```python
from build123d import *

# Parameters (mm, degrees)
SKETCH1_W                                         = 31.75
SKETCH1_H                                         = 160.3375
EXTRUDE1_DEPTH                                    = 62.70625
EXTRUDE2_DEPTH                                    = 107.616906566
EXTRUDE3_REACH                                    = 108.617
SKETCH15_W                                        = 3.96875
SKETCH15_H                                        = 9.525
EXTRUDE6_DEPTH                                    = 173.893618507
CUT_EXTRUDE1_DEPTH                                = 107.616906566
SKETCH17_W                                        = 1.5875
SKETCH17_H                                        = 19.177
CUT_EXTRUDE2_DEPTH                                = 96.8375
CBORE_FOR_1_4_SOCKET_HEAD_CAP_SCREW4_D            = 6.7564
CBORE_FOR_1_4_SOCKET_HEAD_CAP_SCREW4_CBORE_D      = 11.1125
CBORE_FOR_1_4_SOCKET_HEAD_CAP_SCREW4_CBORE_DEPTH  = 6.35
CBORE_FOR_5_16_SOCKET_HEAD_CAP_SCREW2_D           = 8.4328
CBORE_FOR_5_16_SOCKET_HEAD_CAP_SCREW2_DEPTH       = 15.875
CBORE_FOR_5_16_SOCKET_HEAD_CAP_SCREW2_CBORE_D     = 13.49502
CBORE_FOR_5_16_SOCKET_HEAD_CAP_SCREW2_CBORE_DEPTH = 7.9375
CBORE_FOR_5_16_SOCKET_HEAD_CAP_SCREW3_D           = 8.4328
CBORE_FOR_5_16_SOCKET_HEAD_CAP_SCREW3_CBORE_D     = 13.49502
CBORE_FOR_5_16_SOCKET_HEAD_CAP_SCREW3_CBORE_DEPTH = 7.9375
CBORE_FOR_1_4_SOCKET_HEAD_CAP_SCREW2_D            = 6.7564
CBORE_FOR_1_4_SOCKET_HEAD_CAP_SCREW2_CBORE_D      = 11.1125
CBORE_FOR_1_4_SOCKET_HEAD_CAP_SCREW2_CBORE_DEPTH  = 6.35
FILLET1_R                                         = 3.175
SKETCH32_R                                        = 6.35
CUT_EXTRUDE7_DEPTH                                = 22.225
CUT_EXTRUDE8_START                                = 22.225
SKETCH33_R                                        = 6.35
CUT_EXTRUDE8_DEPTH                                = 22.225
SKETCH41_W                                        = 19.05
SKETCH41_H                                        = 25.520262047
CUT_EXTRUDE9_DEPTH                                = 19.05
SKETCH43_W                                        = 6.35
SKETCH43_H                                        = 38.0746
CUT_EXTRUDE11_DEPTH                               = 22.225
CUT_EXTRUDE12_DEPTH                               = 7.14375
CBORE_FOR_1_4_SOCKET_HEAD_CAP_SCREW5_D            = 6.7564
CBORE_FOR_1_4_SOCKET_HEAD_CAP_SCREW5_CBORE_D      = 11.1125
CBORE_FOR_1_4_SOCKET_HEAD_CAP_SCREW5_CBORE_DEPTH  = 9.525
FILLET2_R                                         = 3.175
FILLET3_R                                         = 3.175
CUT_EXTRUDE13_DEPTH                               = 173.893618516
CUT_EXTRUDE14_DEPTH                               = 38.1
FILLET4_R                                         = 3.175


with BuildPart() as part:
    # Sketch1 → Extrude1 (new, symmetric)
    with BuildSketch(Plane.XY):
        Rectangle(SKETCH1_W, SKETCH1_H)
    extrude(amount=EXTRUDE1_DEPTH, both=True)

    # Sketch2 → Extrude2 (cut, through all)
    with BuildSketch(Plane(origin=(15.875, 0, 0), x_dir=(0, 0, -1), z_dir=(1, 0, 0))):
        Polygon((-62.70625, -80.16875), (-61.542285786, -35.71875), (-61.542285786, 80.16875), (-62.70625, 80.16875), align=None)
        Polygon((62.70625, -80.16875), (61.542285786, -35.71875), (61.542285786, 80.16875), (62.70625, 80.16875), align=None)
    extrude(amount=-EXTRUDE2_DEPTH, mode=Mode.SUBTRACT)

    # Sketch3 → Extrude3 (cut, up to next)
    with BuildSketch(Plane(origin=(15.875, 0, 0), x_dir=(0, 0, -1), z_dir=(1, 0, 0)), mode=Mode.PRIVATE) as extrude3_sk1:
        with BuildLine():
            Line((-19.0373, -59.53125), (-19.0373, -50.00625))
            ThreePointArc((-19.0373, -50.00625), (-19.96723597, -47.76118597), (-22.2123, -46.83125))
            Line((-22.2123, -46.83125), (-33.5788, -46.83125))
            ThreePointArc((-33.5788, -46.83125), (-41.5163, -38.89375), (-49.4538, -46.83125))
            Line((-49.4538, -46.83125), (-49.4538, -67.46875))
            ThreePointArc((-49.4538, -67.46875), (-41.5163, -75.40625), (-33.5788, -67.46875))
            Line((-33.5788, -67.46875), (-33.5788, -62.70625))
            Line((-33.5788, -62.70625), (-22.2123, -62.70625))
            ThreePointArc((-22.2123, -62.70625), (-19.96723597, -61.77631403), (-19.0373, -59.53125))
        make_face()
    extrude3_tool1 = extrude(extrude3_sk1.sketch, amount=-EXTRUDE3_REACH, mode=Mode.PRIVATE) & part.part
    # Sketch3 → Extrude3 (cut, up to next)
    with BuildSketch(Plane(origin=(15.875, 0, 0), x_dir=(0, 0, -1), z_dir=(1, 0, 0)), mode=Mode.PRIVATE) as extrude3_sk2:
        with BuildLine():
            Line((49.4538, -67.46875), (49.4538, -46.83125))
            ThreePointArc((49.4538, -46.83125), (41.5163, -38.89375), (33.5788, -46.83125))
            Line((33.5788, -46.83125), (22.2123, -46.83125))
            ThreePointArc((22.2123, -46.83125), (19.96723597, -47.76118597), (19.0373, -50.00625))
            Line((19.0373, -50.00625), (19.0373, -59.53125))
            ThreePointArc((19.0373, -59.53125), (19.96723597, -61.77631403), (22.2123, -62.70625))
            Line((22.2123, -62.70625), (33.5788, -62.70625))
            Line((33.5788, -62.70625), (33.5788, -67.46875))
            ThreePointArc((33.5788, -67.46875), (41.5163, -75.40625), (49.4538, -67.46875))
        make_face()
    extrude3_tool2 = extrude(extrude3_sk2.sketch, amount=-EXTRUDE3_REACH, mode=Mode.PRIVATE) & part.part
    add(extrude3_tool1.solids().sort_by_distance((15.875, -56.432782, 36.973416))[0], mode=Mode.SUBTRACT)
    add(extrude3_tool2.solids().sort_by_distance((15.875, -56.432782, -36.973416))[0], mode=Mode.SUBTRACT)

    # Sketch15 → Extrude6 (cut, through all)
    with BuildSketch(Plane(origin=(0, 80.16875, 0), x_dir=(1, 0, 0), z_dir=(0, 1, 0))):
        with Locations((13.890625, -22.621875)):
            Rectangle(SKETCH15_W, SKETCH15_H)
        with Locations((13.890625, 22.621875)):
            Rectangle(SKETCH15_W, SKETCH15_H)
    extrude(amount=-EXTRUDE6_DEPTH, mode=Mode.SUBTRACT)

    # Sketch16 → Cut-Extrude1 (cut, through all)
    with BuildSketch(Plane(origin=(15.875, 0, 0), x_dir=(0, 0, -1), z_dir=(1, 0, 0))):
        with BuildLine():
            Line((-45.667285786, 80.16875), (45.667285786, 80.16875))
            Line((45.667285786, 80.16875), (45.667285786, -23.01875))
            ThreePointArc((45.667285786, -23.01875), (43.807413847, -27.508878061), (39.317285786, -29.36875))
            Line((39.317285786, -29.36875), (-39.317285786, -29.36875))
            ThreePointArc((-39.317285786, -29.36875), (-43.807413847, -27.508878061), (-45.667285786, -23.01875))
            Line((-45.667285786, -23.01875), (-45.667285786, 80.16875))
        make_face()
    extrude(amount=-CUT_EXTRUDE1_DEPTH, mode=Mode.SUBTRACT)

    # Sketch17 → Cut-Extrude2 (cut, symmetric)
    with BuildSketch(Plane.XY):
        with Locations((-15.08125, -70.58025)):
            Rectangle(SKETCH17_W, SKETCH17_H)
    extrude(amount=CUT_EXTRUDE2_DEPTH, both=True, mode=Mode.SUBTRACT)

    # CBORE for 1/4 Socket Head Cap Screw4 (through all)
    with Locations(Plane(origin=(15.875, 0, 0), x_dir=(0, 0, -1), z_dir=(1, 0, 0))):
        with Locations((-56.35625, -70.58025), (56.35625, -70.58025), (0, -70.58025)):
            CounterBoreHole(CBORE_FOR_1_4_SOCKET_HEAD_CAP_SCREW4_D / 2, CBORE_FOR_1_4_SOCKET_HEAD_CAP_SCREW4_CBORE_D / 2, CBORE_FOR_1_4_SOCKET_HEAD_CAP_SCREW4_CBORE_DEPTH)

    # CBORE for 5/16 Socket Head Cap Screw2
    with Locations(Plane(origin=(0, 0, -61.542285786), x_dir=(-1, 0, 0), z_dir=(0, 0, -1))):
        with Locations((-3.175, 65.88125)):
            CounterBoreHole(CBORE_FOR_5_16_SOCKET_HEAD_CAP_SCREW2_D / 2, CBORE_FOR_5_16_SOCKET_HEAD_CAP_SCREW2_CBORE_D / 2, CBORE_FOR_5_16_SOCKET_HEAD_CAP_SCREW2_CBORE_DEPTH, depth=CBORE_FOR_5_16_SOCKET_HEAD_CAP_SCREW2_DEPTH)

    # CBORE for 5/16 Socket Head Cap Screw3 (through all)
    with Locations(Plane.XY.offset(61.542285786)):
        with Locations((3.175, 65.88125)):
            CounterBoreHole(CBORE_FOR_5_16_SOCKET_HEAD_CAP_SCREW3_D / 2, CBORE_FOR_5_16_SOCKET_HEAD_CAP_SCREW3_CBORE_D / 2, CBORE_FOR_5_16_SOCKET_HEAD_CAP_SCREW3_CBORE_DEPTH)

    # CBORE for 1/4 Socket Head Cap Screw2 (through all)
    with Locations(Plane(origin=(15.875, 0, 0), x_dir=(0, 0, -1), z_dir=(1, 0, 0))):
        with Locations((53.604785786, 48.41875), (-53.604785786, 48.41875)):
            CounterBoreHole(CBORE_FOR_1_4_SOCKET_HEAD_CAP_SCREW2_D / 2, CBORE_FOR_1_4_SOCKET_HEAD_CAP_SCREW2_CBORE_D / 2, CBORE_FOR_1_4_SOCKET_HEAD_CAP_SCREW2_CBORE_DEPTH)

    # Fillet1
    fillet1_edges = [part.edges().sort_by_distance(p)[0] for p in [
        (15.875, -62.70625, -30.4815875),
        (15.875, -62.70625, 30.4815875),
    ]]
    fillet(fillet1_edges, radius=FILLET1_R)

    # Sketch32 → Cut-Extrude7 (cut)
    with BuildSketch(Plane.XY.offset(63.5)):
        with Locations((3.175, -54.76875)):
            Circle(SKETCH32_R)
    extrude(amount=-CUT_EXTRUDE7_DEPTH, mode=Mode.SUBTRACT)

    # Sketch33 → Cut-Extrude8 (cut)
    with BuildSketch(Plane.XY.offset(-63.5).offset(CUT_EXTRUDE8_START)):
        with Locations((3.175, -54.76875)):
            Circle(SKETCH33_R)
    extrude(amount=-CUT_EXTRUDE8_DEPTH, mode=Mode.SUBTRACT)

    # Sketch41 → Cut-Extrude9 (cut)
    with BuildSketch(Plane.ZY.offset(15.875)):
        with Locations((-28.5623, -42.008618977)):
            Rectangle(SKETCH41_W, SKETCH41_H)
        with Locations((28.5623, -42.008618977)):
            Rectangle(SKETCH41_W, SKETCH41_H)
    extrude(amount=-CUT_EXTRUDE9_DEPTH, mode=Mode.SUBTRACT)

    # Sketch43 → Cut-Extrude11 (cut)
    with BuildSketch(Plane(origin=(0, -29.36875, 0), x_dir=(1, 0, 0), z_dir=(0, 1, 0))):
        with Locations((-12.7, 0)):
            Rectangle(SKETCH43_W, SKETCH43_H)
    extrude(amount=-CUT_EXTRUDE11_DEPTH, mode=Mode.SUBTRACT)

    # Sketch44 → Cut-Extrude12 (cut)
    with BuildSketch(Plane.ZY.offset(9.525)):
        with BuildLine():
            Line((-12.7, -29.36875), (12.7, -29.36875))
            Line((12.7, -29.36875), (12.7, -42.8625))
            ThreePointArc((12.7, -42.8625), (11.77006403, -45.10756403), (9.525, -46.0375))
            Line((9.525, -46.0375), (-9.525, -46.0375))
            ThreePointArc((-9.525, -46.0375), (-11.77006403, -45.10756403), (-12.7, -42.8625))
            Line((-12.7, -42.8625), (-12.7, -29.36875))
        make_face()
    extrude(amount=-CUT_EXTRUDE12_DEPTH, mode=Mode.SUBTRACT)

    # CBORE for 1/4 Socket Head Cap Screw5 (through all)
    with Locations(Plane(origin=(15.875, 0, 0), x_dir=(0, 0, -1), z_dir=(1, 0, 0))):
        with Locations((0, -37.30625)):
            CounterBoreHole(CBORE_FOR_1_4_SOCKET_HEAD_CAP_SCREW5_D / 2, CBORE_FOR_1_4_SOCKET_HEAD_CAP_SCREW5_CBORE_D / 2, CBORE_FOR_1_4_SOCKET_HEAD_CAP_SCREW5_CBORE_DEPTH)

    # Fillet2
    # the kernel refuses this fillet: 3.175 mm, written as the material it takes off along each edge
    with BuildSketch(Plane(origin=(15.875, -67.46875, -41.5163), x_dir=(0, 0.842338804567458, 0.5389483633149522), z_dir=(0, 0.5389483633149522, -0.842338804567458))) as fillet2_piece_1:
        with BuildLine():
            CenterArc((7.9375 + FILLET2_R, -FILLET2_R), FILLET2_R, 90, 90)
            Line((7.9375, -FILLET2_R), (7.9375, 0))
            Line((7.9375, 0), (7.9375 + FILLET2_R, 0))
        make_face()
    revolve(axis=Axis((15.875, -67.46875, -41.5163), (1, 0, 0)), revolution_arc=294.775843921, mode=Mode.SUBTRACT)

    # Fillet3
    # the kernel refuses this fillet: 3.175 mm, written as the material it takes off along each edge
    with BuildSketch(Plane(origin=(15.875, -67.46875, 41.5163), x_dir=(0, 0.842338804567458, 0.5389483633149522), z_dir=(0, 0.5389483633149522, -0.842338804567458))) as fillet3_piece_1:
        with BuildLine():
            CenterArc((7.9375 + FILLET3_R, -FILLET3_R), FILLET3_R, 90, 90)
            Line((7.9375, -FILLET3_R), (7.9375, 0))
            Line((7.9375, 0), (7.9375 + FILLET3_R, 0))
        make_face()
    revolve(axis=Axis((15.875, -67.46875, 41.5163), (1, 0, 0)), revolution_arc=294.775843921, mode=Mode.SUBTRACT)

    # Sketch48 → Cut-Extrude13 (cut, through all)
    with BuildSketch(Plane.XZ.offset(80.16875)):
        Polygon((15.875, 0.79375), (15.08125, 0), (15.875, -0.79375), align=None)
    extrude(amount=-CUT_EXTRUDE13_DEPTH, mode=Mode.SUBTRACT)

    # Sketch49 → Cut-Extrude14 (cut, symmetric)
    with BuildSketch(Plane.XY):
        Polygon((15.875, -29.36875), (9.525, -29.36875), (15.875, -35.71875), align=None)
    extrude(amount=CUT_EXTRUDE14_DEPTH, both=True, mode=Mode.SUBTRACT)

    # Fillet4
    fillet4_edges = [part.edges().sort_by_distance(p)[0] for p in [
        (12.7, -32.54375, -38.1),
        (12.7, -32.54375, 38.1),
    ]]
    fillet(fillet4_edges, radius=FILLET4_R)


solid = part.part
```
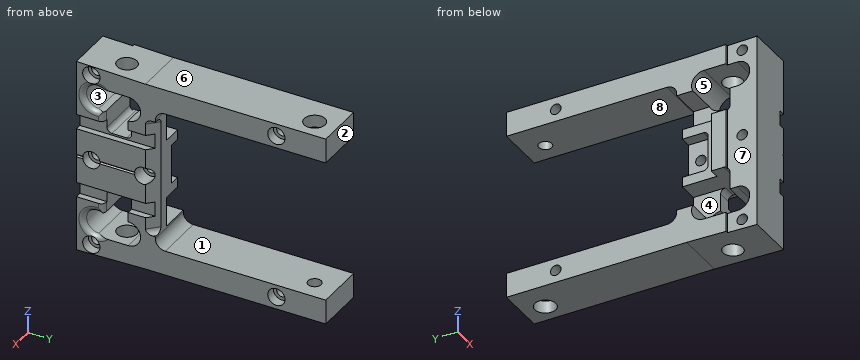
Input: part model. Units: mm. Frame: model coordinates. Face numbers are marked on the shaded views. A direction names the side the tool comes from. Round coordinates to 2 decimals unless told otherwise and drop trailing zeros. Loops run counter-clockwise (first coordinate to the right, second up) from the corner with the lowest first, then second, coordinate; pieces in that order, holes last. Notation, with made-up numbers: (89.25, 31.25) -> (106.25, 31.25) arc R20 ccw to (106.25, 54.25) -> close; hole circle Ø11 at (19, 32.25). An arc over 180 degrees is marked (long way). One line per item, written item: value.
(1) Pin query (flat end, axial travel): pin 1 (16 mm diameter, centred on x = -2, y = 21.5, fed in from +Z); pin 2 (3.5 mm diameter, centred on x = -4.5, z = 2, fed in from +Y); pin 3 (16 mm diameter, centred on x = -5, y = 27.5, fed in from -Z); pin 4 (13 mm diameter, centred on y = 48.42, z = -53.6, fed in from +X) (3 decimals). Return the tip coordinate at first contact, or that it passes through.
Geometry check:
pin 1: z = 61.54
pin 2: y = -46.04
pin 3: z = -61.54
pin 4: x = 15.875
(2) Section B-B (y = -26). Return the cut outline in (x, z) (3 decimals), plus the area to 3 significant figures.
Geometry check:
outline: (-15.875, -61.542) -> (15.875, -61.542) -> (15.875, -44.924) -> (-15.875, -44.924) -> close; (-15.875, 44.924) -> (15.875, 44.924) -> (15.875, 61.542) -> (-15.875, 61.542) -> close
area: 1,060 mm2
(3) Mould query, pull axis Y, two halves, no side actions, for the marked faces 1, 2 and 3. Classes: pulls with the +Y half, pulls with the -Y half, needs draft (parallel to the pull), parting line crosses it, or undercut.
Geometry check:
face 1: needs draft
face 2: pulls with the +Y half
face 3: undercut
(4) Set-up query: the marked faces 4, 5, 6, 7 and 8. Return all of +Z, -Z, +X, -X, +Y, -Y with unobstructed straight access to the full face (end or side cutting, diameter ignored); none if empty.
Geometry check:
face 4: -X, +Y
face 5: +X, -X
face 6: +Z, +X, -X, +Y
face 7: +Z, -Z, -X, -Y
face 8: +X, -X, +Y
(5) Material intervals for line 1 (Z direction, x = -1, y = -7); line 2 (Z direction, x = 10, y = 52); line 3 (Y direction, x = -12.5, z = -54), sorted ascending. Write a range as [from, to].
Geometry check:
line 1: [-61.54, -45.67], [45.67, 61.54]
line 2: [-61.54, -57.85], [-49.36, -45.67], [45.67, 49.36], [57.85, 61.54]
line 3: [-80.17, -73], [-68.16, 45.06], [51.77, 80.17]
(6) Section A-A (y = 37). Return the cut outline in (x, z) (3 decimals), plus the area to 3 significant figures.
Geometry check:
outline: (-15.875, -61.542) -> (15.875, -61.542) -> (15.875, -45.667) -> (-15.875, -45.667) -> close; (-15.875, 45.667) -> (15.875, 45.667) -> (15.875, 61.542) -> (-15.875, 61.542) -> close
area: 1,010 mm2
